Source: CAD feature listing. Evaluate the final solid. Frame: model axes, mm. A direction names the side the tool comes from. Give positions to 0.01 mm unless a question says otherwise; leave off trailing zeros. Order: outer loops, then holes, each group sorted by start corner. A loop starts at its lowest first (then second) coordinate and runs counter-clockwise, first axis right, second up. Notation, with made-up numbers: (9, -10.5) - (30, -10.5) arc R30 cw to (30, 13.5) - close; hole circle Ø10 at (-40, -34). An arc over 180 degrees is marked (long way). Use CSV: the item, a comma, the result in double quotes.
```python
from build123d import *

# Parameters (mm, degrees)
BOSS_EXTRUDE1_DEPTH = 3.175
CHAMFER1_SIZE       = 0.5588
CHAMFER2_SIZE       = 0.5588
CHAMFER2_SIZE_2     = 0.474900858


with BuildPart() as part:
    # Sketch1 → Boss-Extrude1 (new body)
    with BuildSketch(Plane.XY):
        with BuildLine():
            Line((13.884222124, 3.175), (15.878174683, 3.175))
            ThreePointArc((15.878174683, 3.175), (12.996652162, 9.65836885), (7.62, 14.2875))
            Line((7.62, 14.2875), (-7.62, 14.2875))
            ThreePointArc((-7.62, 14.2875), (-12.015852965, 10.854323276), (-14.986, 6.133258534))
            Line((-14.986, 6.133258534), (-14.986, -6.133258534))
            ThreePointArc((-14.986, -6.133258534), (-12.015852965, -10.854323276), (-7.62, -14.2875))
            Line((-7.62, -14.2875), (7.62, -14.2875))
            ThreePointArc((7.62, -14.2875), (12.996652162, -9.65836885), (15.878174683, -3.175))
            Line((15.878174683, -3.175), (13.884222124, -3.175))
            ThreePointArc((13.884222124, -3.175), (-11.1125, 0), (13.884222124, 3.175))
        make_face()
    extrude(amount=BOSS_EXTRUDE1_DEPTH)

    # Chamfer1
    chamfer1_edges = [part.edges().sort_by_distance(p)[0] for p in [
        (-11.1125, 0, 0),
        (-12.015852965, -10.854323276, 0),
        (-12.015852965, 10.854323276, 0),
        (-12.015852965, -10.854323276, 3.175),
        (-11.1125, 0, 3.175),
        (-12.015852965, 10.854323276, 3.175),
    ]]
    chamfer(chamfer1_edges, length=CHAMFER1_SIZE)

    # Chamfer2
    # the kernel refuses this chamfer: 0.5588, 0.474900858 mm, written as the material it takes off along each edge
    with BuildSketch(Plane(origin=(15.878174683, 3.175, -1.437056454), x_dir=(-1, 0, 0), z_dir=(0, 0, 1))) as chamfer2_piece_1:
        with BuildLine():
            Line((CHAMFER2_SIZE, 0), (0.098924499, -0.459875501))
            ThreePointArc((0.098924499, -0.459875501), (0.04906799, -0.236222299), (0, 0))
            Line((0, 0), (CHAMFER2_SIZE, 0))
        make_face()
    extrude(amount=6.049112907, mode=Mode.SUBTRACT)
    with BuildSketch(Plane(origin=(15.878174683, -3.175, -1.413292003), x_dir=(-1, 0, 0), z_dir=(0, 0, 1))) as chamfer2_piece_2:
        with BuildLine():
            Line((CHAMFER2_SIZE_2, 0), (0.116884641, 0.536979589))
            ThreePointArc((0.116884641, 0.536979589), (0.057817387, 0.276572291), (0, 0))
            Line((0, 0), (CHAMFER2_SIZE_2, 0))
        make_face()
    extrude(amount=6.001584006, mode=Mode.SUBTRACT)


solid = part.part
```
Item 1: Material intervals for line 1 (X direction, y = 0, z = 1.9); line 2 (X direction, y = 4.75, z = 1.5); line 3 (Y direction, x = -10, z = 1.05), sorted ascending. Write a range as from..to.
Filled in:
line 1,"x = -14.99..-11.11"
line 2,"x = -14.99..-10.19, 13.37..15.48"
line 3,"y = -12.74..-5.2, 5.2..12.74"
Item 2: Section A-A on z = 2.1. Return the cut outline in (x, y) (1 decimal).
Filled in:
outline,"(-15, -6.1) arc R16.2 ccw to (-7.6, -14.3) - (7.6, -14.3) arc R16.2 ccw to (15.8, -3.7) - (15.4, -3.2) - (13.9, -3.2) arc R12.7 cw (long way) to (13.9, 3.2) - (15.3, 3.2) - (15.8, 3.6) arc R16.2 ccw to (7.6, 14.3) - (-7.6, 14.3) arc R16.2 ccw to (-15, 6.1) - close"
Item 3: Mould query, pull axis X, two halves, no side actions, for faces 1 (the flat face through (-12, 0, 0)), 2 (the cylindrical face through (-11.102, -0.514, 1.573)), 3 (the conical face through (-11.796, 10.49, 0.151)). Classes: released by +X, released by -X, zero draft, split by the parting line, or undercut.
Filled in:
face 1,"zero draft"
face 2,"undercut"
face 3,"released by -X"
Item 4: Set-up query: faces 4 (the conical face through (-11.26, -0.52, 0.4)), 5 (the flat face through (15, -3.175, 2)). Return all of +Z, -Z, +X, -X, +Y, -Y with unobstructed straight access to the full face (end or side cutting, diameter ignored); none if empty.
Filled in:
face 4,"-Z"
face 5,"+Z, -Z, +X"
Item 5: Section B-B on y = 0. Return the cut outline in (x, z) (1 decimal), then the cut area to 3 significant figures.
Filled in:
outline,"(-15, 0) - (-11.7, 0) - (-11.1, 0.6) - (-11.1, 2.6) - (-11.7, 3.2) - (-15, 3.2) - close"
area,"12.0 mm2"
Item 6: First-contact query: pin 1 (1.5 mm diameter, centred on y = -3.5, z = 2, fed in from +X); pin 2 (0.5 mm diameter, centred on x = 14.5, z = 1.5, fed in from +Y); pin 3 (5 mm diameter, centred on x = -8, y = -1.5, fed in from +Z). Flat tips, straight axial feed; report the tip coordinate or a pass-through.
Filled in:
pin 1,"stops at x = 15.76"
pin 2,"stops at y = 7.69"
pin 3,"passes through"
